from build123d import *

# Parameters (mm, degrees)
SKETCH1_W           = 6
SKETCH1_H           = 2.9
BOSS_EXTRUDE1_DEPTH = 4.25
CUT_EXTRUDE1_DEPTH  = 3.2
SKETCH4_W           = 6
SKETCH4_H           = 0.75
CUT_EXTRUDE2_DEPTH  = 0.2
SKETCH5_W           = 0.6
SKETCH5_H           = 0.5
BOSS_EXTRUDE2_DEPTH = 0.85
CUT_EXTRUDE3_DEPTH  = 7.74629528
SKETCH7_W           = 0.3
SKETCH7_H           = 0.5
BOSS_EXTRUDE3_DEPTH = 2.7
CHAMFER1_SIZE       = 0.075
FILLET1_R           = 0.1
CHAMFER2_SIZE       = 0.1


with BuildPart() as part:
    # Sketch1 → Boss-Extrude1 (new body)
    with BuildSketch(Plane(origin=(0, 0, 0), x_dir=(1, 0, 0), z_dir=(0, 1, 0))):
        Rectangle(SKETCH1_W, SKETCH1_H)
    extrude(amount=BOSS_EXTRUDE1_DEPTH)

    # Sketch2 → Cut-Extrude1 (cut)
    with BuildSketch(Plane(origin=(0, 4.25, 0), x_dir=(1, 0, 0), z_dir=(0, 1, 0))):
        Polygon((2.2, 0.04), (2.5, 0.04), (2.5, 0.54), (2.2, 0.54), (2.2, 1.04), (-2.2, 1.04), (-2.2, 0.54), (-2.5, 0.54), (-2.5, 0.04), (-2.2, 0.04), (-2.2, -1.04), (2.2, -1.04), align=None)
    extrude(amount=-CUT_EXTRUDE1_DEPTH, mode=Mode.SUBTRACT)

    # Sketch4 → Cut-Extrude2 (cut)
    with BuildSketch(Plane.XY.offset(1.45)):
        with Locations((0, 0.375)):
            Rectangle(SKETCH4_W, SKETCH4_H)
    extrude(amount=-CUT_EXTRUDE2_DEPTH, mode=Mode.SUBTRACT)

    # Sketch5 → Boss-Extrude2 (add)
    with BuildSketch(Plane.XY.offset(1.25)):
        with Locations((-0.5, 0.25)):
            Rectangle(SKETCH5_W, SKETCH5_H)
        with Locations((-1.5, 0.25)):
            Rectangle(SKETCH5_W, SKETCH5_H)
        with Locations((1.5, 0.25)):
            Rectangle(SKETCH5_W, SKETCH5_H)
        with Locations((0.5, 0.25)):
            Rectangle(SKETCH5_W, SKETCH5_H)
    extrude(amount=BOSS_EXTRUDE2_DEPTH)

    # Sketch6 → Cut-Extrude3 (cut, through all)
    with BuildSketch(Plane(origin=(1.8, 0, 0), x_dir=(0, 0, -1), z_dir=(1, 0, 0))):
        Polygon((-1.35, 0.5), (-1.552072594, 0.15), (-2.1, 0.15), (-2.1, 0.5), align=None)
    extrude(amount=-CUT_EXTRUDE3_DEPTH, mode=Mode.SUBTRACT)

    # Sketch7 → Boss-Extrude3 (add)
    with BuildSketch(Plane(origin=(0, 1.05, 0), x_dir=(1, 0, 0), z_dir=(0, 1, 0))):
        with Locations((-1.5, 0.25)):
            Rectangle(SKETCH7_W, SKETCH7_H)
        with Locations((-0.5, 0.25)):
            Rectangle(SKETCH7_W, SKETCH7_H)
        with Locations((1.5, 0.25)):
            Rectangle(SKETCH7_W, SKETCH7_H)
        with Locations((0.5, 0.25)):
            Rectangle(SKETCH7_W, SKETCH7_H)
    extrude(amount=BOSS_EXTRUDE3_DEPTH)

    # Chamfer1
    chamfer1_edges = [part.edges().sort_by_distance(p)[0] for p in [
        (-0.5, 3.75, 0),
        (-0.65, 3.75, -0.25),
        (-0.5, 3.75, -0.5),
        (-0.35, 3.75, -0.25),
        (-1.5, 3.75, 0),
        (-1.65, 3.75, -0.25),
        (-1.5, 3.75, -0.5),
        (-1.35, 3.75, -0.25),
        (1.5, 3.75, -0.5),
        (1.65, 3.75, -0.25),
        (1.5, 3.75, 0),
        (1.35, 3.75, -0.25),
        (0.35, 3.75, -0.25),
        (0.5, 3.75, -0.5),
        (0.65, 3.75, -0.25),
        (0.5, 3.75, 0),
    ]]
    chamfer(chamfer1_edges, length=CHAMFER1_SIZE)

    # Fillet1
    fillet1_edges = [part.edges().sort_by_distance(p)[0] for p in [
        (0.2, 0.075, 2.1),
        (1.2, 0.075, 2.1),
        (-1.8, 0.075, 2.1),
        (-0.8, 0.075, 2.1),
        (-0.2, 0.075, 2.1),
        (-1.2, 0.075, 2.1),
        (1.8, 0.075, 2.1),
        (0.8, 0.075, 2.1),
    ]]
    fillet(fillet1_edges, radius=FILLET1_R)

    # Chamfer2
    chamfer2_edges = [part.edges().sort_by_distance(p)[0] for p in [
        (2.2, 4.25, -0.79),
        (0, 4.25, -1.04),
        (-2.2, 4.25, -0.79),
        (-2.35, 4.25, -0.54),
        (-2.5, 4.25, -0.29),
        (-2.35, 4.25, -0.04),
        (-2.2, 4.25, 0.5),
        (0, 4.25, 1.04),
        (2.2, 4.25, 0.5),
        (2.35, 4.25, -0.04),
        (2.5, 4.25, -0.29),
        (2.35, 4.25, -0.54),
    ]]
    chamfer(chamfer2_edges, length=CHAMFER2_SIZE)


solid = part.part
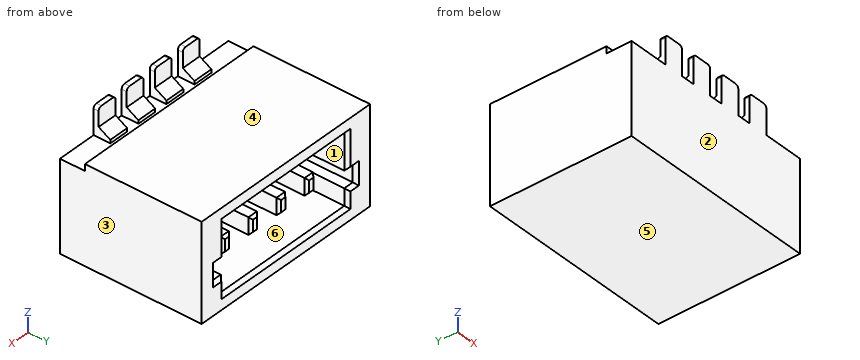
Here's how the part is built. I have some questions about the finished solid (model axes, mm). Face numbers are marked on the shaded views. A direction names the side the tool comes from. Coordinates: 2 decimals unless noted, no trailing zeros. Order: outer loops, then holes, each group sorted by start corner. A loop starts at its lowest first (then second) coordinate and runs counter-clockwise, first axis right, second up. Notation, with made-up numbers: (-1, -0.75) -> (12, -0.75) arc R26 cw to (12, 26.25) -> close; hole circle Ø2 at (-14, 59). An arc over 180 degrees is marked (long way). Answer in a Markdown table with one row per item.
(1) Thinking about a two-plate mould opening in X: for the marked faces 1, 2 and 3, which applies, +X half, -X half, draft (parallel to the pull), parting line (faces both ways), or undercut?
Answer key:
| item | result |
|---|---|
| face 1 | undercut |
| face 2 | draft |
| face 3 | +X half |
(2) On a 3-axis mill with a long thin cutter (end or side, diameter ignored), from which of +Z, -Z, +X, -X, +Y, -Y can I reach the whole of each face in a straight line? I mean the marked faces 4, 5 and 6. Say none if no direction works.
Answer key:
| item | result |
|---|---|
| face 4 | +Z, +X, -X, +Y |
| face 5 | -Z, +X, -X, +Y, -Y |
| face 6 | +Y |
(3) I want a section at B-B on x = -0.5. List the corners of the cut face in (y, z) for me (3 decimals).
Answer key:
| item | result |
|---|---|
| outline | (0, -1.45) -> (4.25, -1.45) -> (4.25, -1.14) -> (4.15, -1.04) -> (1.05, -1.04) -> (1.05, -0.5) -> (3.675, -0.5) -> (3.75, -0.425) -> (3.75, -0.075) -> (3.675, 0) -> (1.05, 0) -> (1.05, 1.04) -> (4.15, 1.04) -> (4.25, 1.14) -> (4.25, 1.45) -> (0.75, 1.45) -> (0.75, 1.25) -> (0.5, 1.25) -> (0.5, 1.35) -> (0.15, 1.552) -> (0.15, 2.1) -> (0, 2.1) -> close |
(4) I want a section at A-A on y = 3.4. Count the separate pieces of the cut face and the enclosed holes in it, then the cut area to 3 significant figures.
Answer key:
| item | result |
|---|---|
| separate pieces | 5 |
| enclosed holes | 1 |
| area | 8.55 mm^2 |
(5) I want a section at C-C on z = 0.2. List the corners of the cut face in (x, y) for me.
Answer key:
| item | result |
|---|---|
| outline | (-3, 0) -> (3, 0) -> (3, 4.25) -> (2.3, 4.25) -> (2.2, 4.15) -> (2.2, 1.05) -> (-2.2, 1.05) -> (-2.2, 4.15) -> (-2.3, 4.25) -> (-3, 4.25) -> close |
(6) I want a section at D-D on y = 0.35. List the corners of the cut face in (x, z) for me.
Answer key:
| item | result |
|---|---|
| outline | (-3, -1.45) -> (3, -1.45) -> (3, 1.25) -> (1.8, 1.25) -> (1.8, 1.44) -> (1.2, 1.44) -> (1.2, 1.25) -> (0.8, 1.25) -> (0.8, 1.44) -> (0.2, 1.44) -> (0.2, 1.25) -> (-0.2, 1.25) -> (-0.2, 1.44) -> (-0.8, 1.44) -> (-0.8, 1.25) -> (-1.2, 1.25) -> (-1.2, 1.44) -> (-1.8, 1.44) -> (-1.8, 1.25) -> (-3, 1.25) -> close |
(7) Please list where these lines run through material, in increasing order: probe 1 along X at (y, z) = (2.3, -0.3); probe 2 along Z at (x, y) = (-0.55, 1.85); probe 3 along X at (y, z) = (3.1, -0.7).
Answer key:
| item | result |
|---|---|
| probe 1 | -3 to -2.5, -1.65 to -1.35, -0.65 to -0.35, 0.35 to 0.65, 1.35 to 1.65, 2.5 to 3 |
| probe 2 | -1.45 to -1.04, -0.5 to 0, 1.04 to 1.45 |
| probe 3 | -3 to -2.2, 2.2 to 3 |
(8) Will this pin go through, and if not, where does the flat tip stop? pin 1 Ø2 at (x, z) = (2, -0.5) entering from +Y.
Answer key:
| item | result |
|---|---|
| pin 1 | y = 4.25 |
